Could you check a few things on this model? Use its own coordinates, in mm. Face numbers are marked on the shaded views. A direction names the side the tool comes from. Round coordinates to 2 decimals unless told otherwise and drop trailing zeros. Write each loop counter-clockwise with the first axis right and the second up, starting at its lowest first coordinate (ties: lowest second). Pieces come first, ordered by that corner, then holes. Notation, with made-up numbers: (-21, -6.5) -> (17, -6.5) arc R23 ccw to (17, 14.5) -> close; hole circle Ø8 at (9.5, -38). An arc over 180 degrees is marked (long way). Answer in a Markdown table with one row per item.
from build123d import *

# Parameters (mm, degrees)
SKETCH_1_R          = 27.5
EXTRUDE_1_DEPTH     = 3
SKETCH_2_R          = 22.5
EXTRUDE_2_DEPTH     = 10
CUT_EXTRUDE_1_REACH = 43.006
SKETCH_3_R          = 1.7
SKETCH_3_R_2        = 4
EXTRUDE_3_DEPTH     = 7
SKETCH_6_R          = 3
CUT_EXTRUDE_2_DEPTH = 3
CUT_EXTRUDE_3_REACH = 62
SKETCH_7_R          = 2.5


with BuildPart() as part:
    # 草图1 → 凸台-拉伸1 (new body)
    with BuildSketch(Plane(origin=(0, 0, 0), x_dir=(1, 0, 0), z_dir=(0, 1, 0))):
        with Locations(Location((0, 0, 0), (0, 0, 270))):
            Circle(SKETCH_1_R)
    extrude(amount=-EXTRUDE_1_DEPTH)

    # 草图2 → 凸台-拉伸2 (add)
    with BuildSketch(Plane.XZ.offset(3)):
        with Locations(Location((0, 0, 0), (0, 0, 270))):
            Circle(SKETCH_2_R)
    extrude(amount=EXTRUDE_2_DEPTH)

    # 草图3 → 切除-拉伸1 (cut, up to next)
    with BuildSketch(Plane.XZ.offset(13), mode=Mode.PRIVATE) as cut_extrude_1_sk1:
        with Locations(Location((0, 17.5, 0), (0, 0, 270))):
            Circle(SKETCH_3_R)
    cut_extrude_1_tool1 = extrude(cut_extrude_1_sk1.sketch, amount=-CUT_EXTRUDE_1_REACH, mode=Mode.PRIVATE) & part.part
    # 草图3 → 切除-拉伸1 (cut, up to next)
    with BuildSketch(Plane.XZ.offset(13), mode=Mode.PRIVATE) as cut_extrude_1_sk2:
        with Locations(Location((17.5, 0, 0), (0, 0, 270))):
            Circle(SKETCH_3_R)
    cut_extrude_1_tool2 = extrude(cut_extrude_1_sk2.sketch, amount=-CUT_EXTRUDE_1_REACH, mode=Mode.PRIVATE) & part.part
    # 草图3 → 切除-拉伸1 (cut, up to next)
    with BuildSketch(Plane.XZ.offset(13), mode=Mode.PRIVATE) as cut_extrude_1_sk3:
        with Locations(Location((0, -17.5, 0), (0, 0, 270))):
            Circle(SKETCH_3_R)
    cut_extrude_1_tool3 = extrude(cut_extrude_1_sk3.sketch, amount=-CUT_EXTRUDE_1_REACH, mode=Mode.PRIVATE) & part.part
    # 草图3 → 切除-拉伸1 (cut, up to next)
    with BuildSketch(Plane.XZ.offset(13), mode=Mode.PRIVATE) as cut_extrude_1_sk4:
        with Locations(Location((-17.5, 0, 0), (0, 0, 270))):
            Circle(SKETCH_3_R)
    cut_extrude_1_tool4 = extrude(cut_extrude_1_sk4.sketch, amount=-CUT_EXTRUDE_1_REACH, mode=Mode.PRIVATE) & part.part
    # 草图3 → 切除-拉伸1 (cut, up to next)
    with BuildSketch(Plane.XZ.offset(13), mode=Mode.PRIVATE) as cut_extrude_1_sk5:
        with Locations(Location((0, 0, 0), (0, 0, 270))):
            Circle(SKETCH_3_R_2)
    cut_extrude_1_tool5 = extrude(cut_extrude_1_sk5.sketch, amount=-CUT_EXTRUDE_1_REACH, mode=Mode.PRIVATE) & part.part
    add(cut_extrude_1_tool1.solids().sort_by_distance((0, -13, 17.5))[0], mode=Mode.SUBTRACT)
    add(cut_extrude_1_tool2.solids().sort_by_distance((17.5, -13, 0))[0], mode=Mode.SUBTRACT)
    add(cut_extrude_1_tool3.solids().sort_by_distance((0, -13, -17.5))[0], mode=Mode.SUBTRACT)
    add(cut_extrude_1_tool4.solids().sort_by_distance((-17.5, -13, 0))[0], mode=Mode.SUBTRACT)
    add(cut_extrude_1_tool5.solids().sort_by_distance((0, -13, 0))[0], mode=Mode.SUBTRACT)

    # 草图4 → 凸台-拉伸3 (add)
    with BuildSketch(Plane(origin=(0, 0, 0), x_dir=(1, 0, 0), z_dir=(0, 1, 0))):
        Polygon((0, 40), (16.568542495, 40), (40, 16.568542495), (40, 0), (40, -16.568542495), (16.568542495, -40), (0, -40), (-16.568542495, -40), (-40, -16.568542495), (-40, 0), (-40, 16.568542495), (-16.568542495, 40), align=None)
        Polygon((0, 21.5), (3.248737342, 21.5), (21.5, 3.248737342), (21.5, 0), (21.5, -3.248737342), (3.248737342, -21.5), (0, -21.5), (-3.248737342, -21.5), (-21.5, -3.248737342), (-21.5, 0), (-21.5, 3.248737342), (-3.248737342, 21.5), align=None, mode=Mode.SUBTRACT)
    extrude(amount=EXTRUDE_3_DEPTH)

    # 草图6 → 切除-拉伸2 (cut)
    with BuildSketch(Plane(origin=(0, 7, 0), x_dir=(1, 0, 0), z_dir=(0, 1, 0))):
        with Locations(Location((20.859650045, 20.859650045, 0), (0, 0, 270))):
            Circle(SKETCH_6_R)
        with Locations(Location((20.859650045, -20.859650045, 0), (0, 0, 270))):
            Circle(SKETCH_6_R)
        with Locations(Location((-20.859650045, -20.859650045, 0), (0, 0, 270))):
            Circle(SKETCH_6_R)
        with Locations(Location((-20.859650045, 20.859650045, 0), (0, 0, 270))):
            Circle(SKETCH_6_R)
    extrude(amount=-CUT_EXTRUDE_2_DEPTH, mode=Mode.SUBTRACT)

    # 草图7 → 切除-拉伸3 (cut, up to next)
    with BuildSketch(Plane(origin=(0, 7, 0), x_dir=(1, 0, 0), z_dir=(0, 1, 0)), mode=Mode.PRIVATE) as cut_extrude_3_sk1:
        with Locations(Location((9.545941546, 32.173358544, 0), (0, 0, 270))):
            Circle(SKETCH_7_R)
    cut_extrude_3_tool1 = extrude(cut_extrude_3_sk1.sketch, amount=-CUT_EXTRUDE_3_REACH, mode=Mode.PRIVATE) & part.part
    # 草图7 → 切除-拉伸3 (cut, up to next)
    with BuildSketch(Plane(origin=(0, 7, 0), x_dir=(1, 0, 0), z_dir=(0, 1, 0)), mode=Mode.PRIVATE) as cut_extrude_3_sk2:
        with Locations(Location((32.173358544, 9.545941546, 0), (0, 0, 270))):
            Circle(SKETCH_7_R)
    cut_extrude_3_tool2 = extrude(cut_extrude_3_sk2.sketch, amount=-CUT_EXTRUDE_3_REACH, mode=Mode.PRIVATE) & part.part
    # 草图7 → 切除-拉伸3 (cut, up to next)
    with BuildSketch(Plane(origin=(0, 7, 0), x_dir=(1, 0, 0), z_dir=(0, 1, 0)), mode=Mode.PRIVATE) as cut_extrude_3_sk3:
        with Locations(Location((32.173358544, -9.545941546, 0), (0, 0, 270))):
            Circle(SKETCH_7_R)
    cut_extrude_3_tool3 = extrude(cut_extrude_3_sk3.sketch, amount=-CUT_EXTRUDE_3_REACH, mode=Mode.PRIVATE) & part.part
    # 草图7 → 切除-拉伸3 (cut, up to next)
    with BuildSketch(Plane(origin=(0, 7, 0), x_dir=(1, 0, 0), z_dir=(0, 1, 0)), mode=Mode.PRIVATE) as cut_extrude_3_sk4:
        with Locations(Location((9.545941546, -32.173358544, 0), (0, 0, 270))):
            Circle(SKETCH_7_R)
    cut_extrude_3_tool4 = extrude(cut_extrude_3_sk4.sketch, amount=-CUT_EXTRUDE_3_REACH, mode=Mode.PRIVATE) & part.part
    # 草图7 → 切除-拉伸3 (cut, up to next)
    with BuildSketch(Plane(origin=(0, 7, 0), x_dir=(1, 0, 0), z_dir=(0, 1, 0)), mode=Mode.PRIVATE) as cut_extrude_3_sk5:
        with Locations(Location((-9.545941546, -32.173358544, 0), (0, 0, 270))):
            Circle(SKETCH_7_R)
    cut_extrude_3_tool5 = extrude(cut_extrude_3_sk5.sketch, amount=-CUT_EXTRUDE_3_REACH, mode=Mode.PRIVATE) & part.part
    # 草图7 → 切除-拉伸3 (cut, up to next)
    with BuildSketch(Plane(origin=(0, 7, 0), x_dir=(1, 0, 0), z_dir=(0, 1, 0)), mode=Mode.PRIVATE) as cut_extrude_3_sk6:
        with Locations(Location((-32.173358544, -9.545941546, 0), (0, 0, 270))):
            Circle(SKETCH_7_R)
    cut_extrude_3_tool6 = extrude(cut_extrude_3_sk6.sketch, amount=-CUT_EXTRUDE_3_REACH, mode=Mode.PRIVATE) & part.part
    # 草图7 → 切除-拉伸3 (cut, up to next)
    with BuildSketch(Plane(origin=(0, 7, 0), x_dir=(1, 0, 0), z_dir=(0, 1, 0)), mode=Mode.PRIVATE) as cut_extrude_3_sk7:
        with Locations(Location((-32.173358544, 9.545941546, 0), (0, 0, 270))):
            Circle(SKETCH_7_R)
    cut_extrude_3_tool7 = extrude(cut_extrude_3_sk7.sketch, amount=-CUT_EXTRUDE_3_REACH, mode=Mode.PRIVATE) & part.part
    # 草图7 → 切除-拉伸3 (cut, up to next)
    with BuildSketch(Plane(origin=(0, 7, 0), x_dir=(1, 0, 0), z_dir=(0, 1, 0)), mode=Mode.PRIVATE) as cut_extrude_3_sk8:
        with Locations(Location((-9.545941546, 32.173358544, 0), (0, 0, 270))):
            Circle(SKETCH_7_R)
    cut_extrude_3_tool8 = extrude(cut_extrude_3_sk8.sketch, amount=-CUT_EXTRUDE_3_REACH, mode=Mode.PRIVATE) & part.part
    add(cut_extrude_3_tool1.solids().sort_by_distance((9.545942, 7, -32.173359))[0], mode=Mode.SUBTRACT)
    add(cut_extrude_3_tool2.solids().sort_by_distance((32.173359, 7, -9.545942))[0], mode=Mode.SUBTRACT)
    add(cut_extrude_3_tool3.solids().sort_by_distance((32.173359, 7, 9.545942))[0], mode=Mode.SUBTRACT)
    add(cut_extrude_3_tool4.solids().sort_by_distance((9.545942, 7, 32.173359))[0], mode=Mode.SUBTRACT)
    add(cut_extrude_3_tool5.solids().sort_by_distance((-9.545942, 7, 32.173359))[0], mode=Mode.SUBTRACT)
    add(cut_extrude_3_tool6.solids().sort_by_distance((-32.173359, 7, 9.545942))[0], mode=Mode.SUBTRACT)
    add(cut_extrude_3_tool7.solids().sort_by_distance((-32.173359, 7, -9.545942))[0], mode=Mode.SUBTRACT)
    add(cut_extrude_3_tool8.solids().sort_by_distance((-9.545942, 7, -32.173359))[0], mode=Mode.SUBTRACT)


solid = part.part
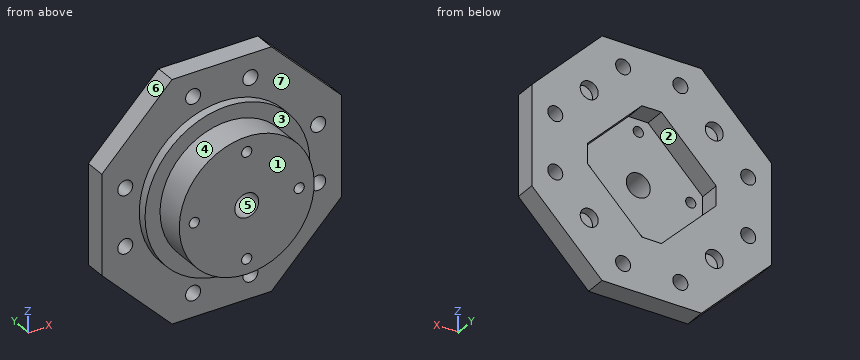
1) For the marked faces 1, 2 and 3, which set-ups out of +Z, -Z, +X, -X, +Y, -Y let a thin tool reach every point of the face, with its end or its side?
Findings:
| item | result |
|---|---|
| face 1 | +Z, -Z, +X, -X, -Y |
| face 2 | +Y |
| face 3 | -Y |
2) Thinking about a two-plate mould opening in X: for the marked faces 4, 5, 6 and 7, which applies, +X half, -X half, draft (parallel to the pull), parting line (faces both ways), or undercut?
Findings:
| item | result |
|---|---|
| face 4 | parting line |
| face 5 | undercut |
| face 6 | -X half |
| face 7 | draft |
3) Imagine slicing it at D-D, the plane z = 8. Please give me the cut outline in (x, y), plus the area to 3 significant figures.
Findings:
| item | result |
|---|---|
| outline | (-40, 0) -> (-34.14, 0) -> (-34.14, 7) -> (-40, 7) -> close; (-30.21, 0) -> (-26.31, 0) -> (-26.31, -3) -> (-21.03, -3) -> (-21.03, -13) -> (21.03, -13) -> (21.03, -3) -> (26.31, -3) -> (26.31, 0) -> (30.21, 0) -> (30.21, 7) -> (16.75, 7) -> (16.75, 0) -> (-16.75, 0) -> (-16.75, 7) -> (-30.21, 7) -> close; (34.14, 0) -> (40, 0) -> (40, 7) -> (34.14, 7) -> close |
| area | 849 mm^2 |
4) Please list where these lines run through material, in increasing order: line 1 (Z direction, x = -3, y = 4.5); line 2 (X direction, y = 1, z = -31.5); line 3 (Z direction, x = 32, y = 0.75).
Findings:
| item | result |
|---|---|
| line 1 | z = -40 to -21.5, 21.5 to 40 |
| line 2 | x = -25.07 to -11.95, -7.14 to 7.14, 11.95 to 25.07 |
| line 3 | z = -24.57 to -12.04, -7.05 to 7.05, 12.04 to 24.57 |
5) For pin 1 (5.5 mm diameter, centred on x = -20.86, z = -20.86, fed in from +Y); pin 2 (21.5 mm diameter, centred on x = -4, z = 2, fed in from +Y); pin 3 (4 mm diameter, centred on x = 18.5, z = -25, fed in from -Y), each with a flat end and sliding along its axis, tell me the tip position at first contact or that it passes through.
Findings:
| item | result |
|---|---|
| pin 1 | stops at y = 4 |
| pin 2 | stops at y = 0 |
| pin 3 | stops at y = 0 |
6) Imagine slicing it at A-A, the plane x = 0. Please give me the cut outline in (y, z).
Findings:
| item | result |
|---|---|
| outline | (-13, -22.5) -> (-3, -22.5) -> (-3, -27.5) -> (0, -27.5) -> (0, -40) -> (7, -40) -> (7, -21.5) -> (0, -21.5) -> (0, -19.2) -> (-13, -19.2) -> close; (-13, -15.8) -> (0, -15.8) -> (0, -4) -> (-13, -4) -> close; (-13, 4) -> (0, 4) -> (0, 15.8) -> (-13, 15.8) -> close; (-13, 19.2) -> (0, 19.2) -> (0, 21.5) -> (7, 21.5) -> (7, 40) -> (0, 40) -> (0, 27.5) -> (-3, 27.5) -> (-3, 22.5) -> (-13, 22.5) -> close |
7) Imagine slicing it at C-C, the plane y = -7.75. Please give me the cut outline in (x, z), plus the area to 3 significant figures.
Findings:
| item | result |
|---|---|
| outline | circle Ø45 at (0, 0); hole circle Ø3.4 at (-17.5, 0); hole circle Ø8 at (0, 0); hole circle Ø3.4 at (0, -17.5); hole circle Ø3.4 at (0, 17.5); hole circle Ø3.4 at (17.5, 0) |
| area | 1,500 mm^2 |
8) Imagine slicing it at B-B, the plane z = 0. Please give me the cut outline in (x, y), plus the area to 3 significant figures.
Findings:
| item | result |
|---|---|
| outline | (-40, 0) -> (-27.5, 0) -> (-27.5, -3) -> (-22.5, -3) -> (-22.5, -13) -> (-19.2, -13) -> (-19.2, 0) -> (-21.5, 0) -> (-21.5, 7) -> (-40, 7) -> close; (-15.8, -13) -> (-4, -13) -> (-4, 0) -> (-15.8, 0) -> close; (4, -13) -> (15.8, -13) -> (15.8, 0) -> (4, 0) -> close; (19.2, -13) -> (22.5, -13) -> (22.5, -3) -> (27.5, -3) -> (27.5, 0) -> (40, 0) -> (40, 7) -> (21.5, 7) -> (21.5, 0) -> (19.2, 0) -> close |
| area | 682 mm^2 |
